Input: part model. Units: mm. Frame: model coordinates. Face numbers are marked on the shaded views. A direction names the side the tool comes from. Coordinates: 2 decimals unless noted, no trailing zeros. Order: outer loops, then holes, each group sorted by start corner. A loop starts at its lowest first (then second) coordinate and runs counter-clockwise, first axis right, second up. Notation, with made-up numbers: (-26, 6) -> (-11, 6) arc R25 cw to (-11, 44) -> close; hole circle Ø2 at (4.25, 13). An arc over 180 degrees is marked (long way). Use one line per item in the form item = value. Start each with the question number.
1) Section query B-B on x = 42.5. Output: boundary loops of the cut face in (y, z), then the cut area to 3 significant figures.
2) Access query for the marked faces 4, 5 and 6. Directions: +Z, -Z, +X, -X, +Y, -Y. A direction counts if a zero-diameter tool reaches every point of the face in a straight line with its end or side. Return the directions, or none.
3) Section query D-D on z = -3. Output: boundary loops of the cut face in (x, y), then the cut area to 3 significant figures.
4) Pin query (flat end, axial travel): pin 1 (5 mm diameter, centred on x = -10, y = 11.75, fed in from -Z); pin 2 (1.5 mm diameter, centred on y = 24.5, z = -34.5, fed in from -X); pin 3 (4.5 mm diameter, centred on y = 4.5, z = -18, fed in from -X). Return the tip coordinate at first contact, or that it passes through.
5) Draft query along X for the marked faces 1, 2 and 3. Return one class per face: pulls with the +X half, pulls with the -X half, needs draft (parallel to the pull), parting line crosses it, or undercut.
6) Section query C-C on z = 9. Output: boundary loops of the cut face in (x, y), then the cut area to 3 significant figures.
7) Section query A-A on z = -17. Output: boundary loops of the cut face in (x, y), then the cut area to 3 significant figures.
8) Ray query, line 1 along X through (y, z) = (27.5, -21); line 2 along Y through (x, z) = (37.95, -16.25); line 3 along Y through (x, z) = (49, -5.5). Return the intervals inside material, ascending.
from build123d import *

# Parameters (mm, degrees)
SKETCH2_R                = 22
SKETCH2_W                = 16.20928
SKETCH2_H                = 20.5
BOSS_EXTRUDE1_DEPTH      = 2
SKETCH6_R                = 2
BOSS_EXTRUDE3_DEPTH      = 5.6
SKETCH7_R                = 2.739
BOSS_EXTRUDE4_DEPTH      = 4
BOSS_EXTRUDE5_DEPTH      = 5
BOSS_EXTRUDE5_DEPTH_BACK = 3.5
SKETCH9_R                = 2
LOFT4_START              = -19.749341788
LOFT4_DEPTH              = 14.749341788
LOFT4_START_2            = 11
LOFT4_2_DEPTH            = 20
CUT_EXTRUDE1_START       = -5
SKETCH11_R               = 3.81
CUT_EXTRUDE1_DEPTH       = 5
CUT_EXTRUDE2_REACH       = 99.148
SKETCH12_R               = 3
BOSS_EXTRUDE9_DEPTH      = 4
SKETCH14_R               = 1.9
CUT_EXTRUDE3_DEPTH       = 86.385585859
CUT_EXTRUDE5_START       = -5
CUT_EXTRUDE5_DEPTH       = 5


with BuildPart() as part:
    # Sketch2 → Boss-Extrude1 (new body)
    with BuildSketch(Plane(origin=(0, 0, 0), x_dir=(1, 0, 0), z_dir=(0, 1, 0))):
        with BuildLine():
            Line((35.10955, 44.5), (-7.045717951, 36.322965993))
            ThreePointArc((-7.045717951, 36.322965993), (-21.445207215, 30.151336413), (-32, 18.574175621))
            Line((-32, 18.574175621), (-32, -18.574175621))
            ThreePointArc((-32, -18.574175621), (-3.042934445, -36.874659998), (28.522340191, -23.568540685))
            Line((28.522340191, -23.568540685), (56.860578118, 10.726024828))
            ThreePointArc((56.860578118, 10.726024828), (57.200783272, 11.323056958), (57.31883, 12))
            Line((57.31883, 12), (57.31883, 32.5))
            ThreePointArc((57.31883, 32.5), (57.058008676, 33.487551282), (56.343572466, 34.21752813))
            Line((56.343572466, 34.21752813), (39.10955, 44.5))
            Line((39.10955, 44.5), (35.10955, 44.5))
        make_face()
        with Locations(Location((0, 0, 0), (0, 0, 270))):
            Circle(SKETCH2_R, mode=Mode.SUBTRACT)
        with Locations((47.21419, 22.25)):
            Rectangle(SKETCH2_W, SKETCH2_H, mode=Mode.SUBTRACT)
    extrude(amount=-BOSS_EXTRUDE1_DEPTH)

    # Sketch6 → Boss-Extrude3 (add)
    with BuildSketch(Plane.XY.offset(-14.45)):
        Polygon((23.512808221, 0), (23.512808221, 8.5), (30.35955, 17.5), (35.10955, 17.5), (35.10955, 0), align=None)
        with Locations((29.22955, 11)):
            Circle(SKETCH6_R, mode=Mode.SUBTRACT)
    extrude(amount=-BOSS_EXTRUDE3_DEPTH)

    # Sketch7 → Boss-Extrude4 (add)
    with BuildSketch(Plane(origin=(35.10955, 0, 0), x_dir=(0, 0, -1), z_dir=(1, 0, 0))):
        Polygon((44.5, 0), (10.25, 0), (10.25, 49), (23.5, 49), align=None)
        with Locations((16.25, 43)):
            Circle(SKETCH7_R, mode=Mode.SUBTRACT)
    extrude(amount=BOSS_EXTRUDE4_DEPTH)



with BuildPart() as body_2:
    # Sketch9 → Boss-Extrude5 (new, two sides: drawn at the far end of the back side and taken through both)
    with BuildSketch(Plane.XY.offset(15.5).offset(-BOSS_EXTRUDE5_DEPTH_BACK)):
        with BuildLine():
            Line((-15, 11.75), (-15, 6.75))
            Line((-15, 6.75), (-10, 6.75))
            Line((-10, 6.75), (-5, 6.75))
            Line((-5, 6.75), (-5, 11.75))
            ThreePointArc((-5, 11.75), (-10, 16.75), (-15, 11.75))
        make_face()
        with Locations((-10, 11.75)):
            Circle(SKETCH9_R, mode=Mode.SUBTRACT)
    extrude(amount=BOSS_EXTRUDE5_DEPTH + BOSS_EXTRUDE5_DEPTH_BACK)


with BuildPart() as part_1:
    add(part.part)

    add(body_2.part)  # Loft4 merges body 2
    # Loft4: read off the stored shape, not the designer's step
    # Loft4 outline → Loft4 (add)
    with BuildSketch(Plane.YZ.offset(LOFT4_START)):
        Polygon((6.75, 20.5), (0, 29.981530337), (0, 21.424285286), (6.75, 12), align=None)
    extrude(amount=LOFT4_DEPTH)

    # Loft4 2 outline → Loft4 2 (cut)
    with BuildSketch(Plane.XY.offset(LOFT4_START_2)):
        Polygon((-19.749341788, 0), (-15, 6.75), (-19.749341788, 6.75), align=None)
    extrude(amount=LOFT4_2_DEPTH, mode=Mode.SUBTRACT)

    # Sketch11 → Cut-Extrude1 (cut)
    with BuildSketch(Plane.XY.offset(20.5).offset(CUT_EXTRUDE1_START)):
        with Locations((-10, 11.75)):
            Circle(SKETCH11_R)
    extrude(amount=CUT_EXTRUDE1_DEPTH, mode=Mode.SUBTRACT)

    # Sketch13 → Cut-Extrude2 (cut, up to next)
    with BuildSketch(Plane(origin=(39.10955, 0, 0), x_dir=(0, 0, -1), z_dir=(1, 0, 0)), mode=Mode.PRIVATE) as cut_extrude2_sk1:
        Polygon((44.5, 0), (38.5, 0), (38.5, 14), align=None)
    cut_extrude2_tool1 = extrude(cut_extrude2_sk1.sketch, amount=-CUT_EXTRUDE2_REACH, mode=Mode.PRIVATE) & part_1.part
    add(cut_extrude2_tool1.solids().sort_by_distance((39.10955, 4.666667, -40.5))[0], mode=Mode.SUBTRACT)

    # Sketch12 → Boss-Extrude9 (add)
    with BuildSketch(Plane(origin=(0, 0, 0), x_dir=(1, 0, 0), z_dir=(0, 1, 0))):
        with Locations(Location((-24.04163056, 24.04163056, 0), (0, 0, 134.999512051))):
            Circle(SKETCH12_R)
        with Locations(Location((-24.04163056, -24.04163056, 0), (0, 0, 224.999512051))):
            Circle(SKETCH12_R)
        with Locations(Location((24.04163056, -24.04163056, 0), (0, 0, 314.999512068))):
            Circle(SKETCH12_R)
        with Locations(Location((47.21419, 3.761759805, 0), (0, 0, 320.432443614))):
            Circle(SKETCH12_R)
        with Locations((35.10955, 41.444082154)):
            Circle(SKETCH12_R)
    extrude(amount=BOSS_EXTRUDE9_DEPTH)

    # Sketch14 → Cut-Extrude3 (cut, through all)
    with BuildSketch(Plane(origin=(0, 4, 0), x_dir=(1, 0, 0), z_dir=(0, 1, 0))):
        with Locations(Location((-24.04163056, 24.04163056, 0), (0, 0, 270))):
            Circle(SKETCH14_R)
        with Locations(Location((35.10955, 41.444082154, 0), (0, 0, 270))):
            Circle(SKETCH14_R)
        with Locations(Location((47.21419, 3.761759805, 0), (0, 0, 270))):
            Circle(SKETCH14_R)
        with Locations(Location((24.04163056, -24.04163056, 0), (0, 0, 270))):
            Circle(SKETCH14_R)
        with Locations(Location((-24.04163056, -24.04163056, 0), (0, 0, 270))):
            Circle(SKETCH14_R)
    extrude(amount=-CUT_EXTRUDE3_DEPTH, mode=Mode.SUBTRACT)

    # Sketch18 → Cut-Extrude5 (cut)
    with BuildSketch(Plane.XY.offset(20.5).offset(CUT_EXTRUDE5_START)):
        with BuildLine():
            Line((-10, 11.75), (-12.694076836, 14.444076836))
            Line((-12.694076836, 14.444076836), (-14.212119419, 14.444076836))
            ThreePointArc((-14.212119419, 14.444076836), (-10, 16.75), (-5.787880581, 14.444076836))
            Line((-5.787880581, 14.444076836), (-7.305923164, 14.444076836))
            Line((-7.305923164, 14.444076836), (-10, 11.75))
        make_face()
    extrude(amount=CUT_EXTRUDE5_DEPTH, mode=Mode.SUBTRACT)


solid = part_1.part
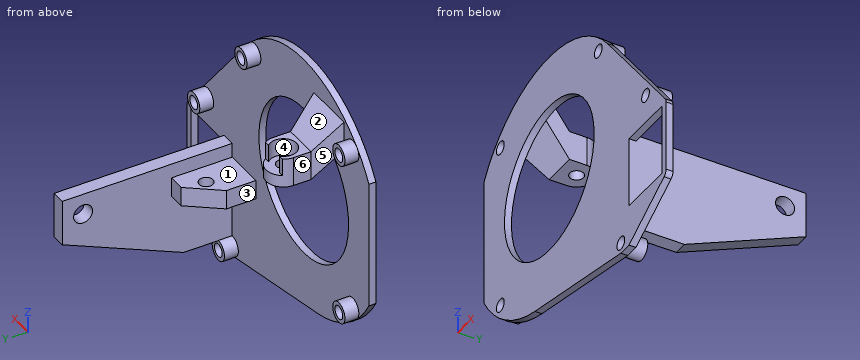
Answers below:
q1.outline = (-2, -42.48) -> (0, -42.48) -> (0, -32.5) -> (-2, -32.5) -> close; (-2, -12) -> (0, -12) -> (0, 6.65) -> (-2, 6.65) -> close
q1.area = 57.3 mm^2
q2.face_4 = +Z
q2.face_5 = +Z, -Z, +Y
q2.face_6 = +Z, -Z, -X, +Y
q3.outline = (-32, -2) -> (-21.79, -2) -> (-21.79, 0) -> (-32, 0) -> close; (21.79, -2) -> (45.47, -2) -> (45.47, 4) -> (44.31, 4) -> (44.31, 0) -> (21.79, 0) -> close; (48.95, -2) -> (50.48, -2) -> (50.48, 0) -> (50.12, 0) -> (50.12, 4) -> (48.95, 4) -> close
q3.area = 80.1 mm^2
q4.pin_1 = 12
q4.pin_2 = 35.11
q4.pin_3 = 23.51
q5.face_1 = needs draft
q5.face_2 = undercut
q5.face_3 = pulls with the -X half
q6.outline = (-32, -2) -> (-20.07, -2) -> (-20.07, 0) -> (-32, 0) -> close; (20.07, -2) -> (40.56, -2) -> (40.56, 0) -> (20.07, 0) -> close
q6.area = 64.8 mm^2
q7.outline = (-32, -2) -> (-13.96, -2) -> (-13.96, 0) -> (-32, 0) -> close; (13.96, -2) -> (39.11, -2) -> (39.11, 40.37) -> (35.11, 40.37) -> (35.11, 17.5) -> (30.36, 17.5) -> (23.51, 8.5) -> (23.51, 0) -> (13.96, 0) -> close; (35.11, 45.63) -> (39.11, 45.63) -> (39.11, 49) -> (35.11, 49) -> close; (55.32, -2) -> (57.32, -2) -> (57.32, 0) -> (55.32, 0) -> close; hole circle Ø4 at (29.23, 11)
q7.area = 425 mm^2
q8.line_1 = 35.11 to 39.11
q8.line_2 = -2 to 40.26, 45.74 to 49
q8.line_3 = -2 to 4
